Model file for the job. Use its own axes, mm. Face numbers are marked on the shaded views. A direction names the side the tool comes from. Coordinates: 2 decimals unless noted, no trailing zeros. Answer as a JSON object with one key per item and string values. Group by question number.
from build123d import *

# Parameters (mm, degrees)
F0_R     = 11
F1_DEPTH = 7
F2_R     = 3.4999


# Not quite as in the source:
# - a fillet or chamfer is up to 0.001 mm smaller than in the source, because OpenCascade refuses the exact size


with BuildPart() as f1:
    # F0 (on Front) → F1 (new body)
    with BuildSketch(Plane.XZ):
        with BuildLine():
            add(Edge.make_bspline(
                [(0, 31.75), (-29.1176115239, 31.75), (-14.558805762, -15.875), (0, -63.5), (14.558805762, -15.875), (29.1176115239, 31.75), (0, 31.75)],
                knots=[0, 0, 0, 2.0943951024, 2.0943951024, 4.1887902048, 4.1887902048, 6.2831853072, 6.2831853072, 6.2831853072], degree=2, weights=[1, 0.5, 1, 0.5, 1, 0.5, 1]))
        make_face()
        Polygon((2.9989406364, -15.1111775695), (6.0104428668, -20.3127475603), (3.0115022304, -25.5215699908), (-2.9989406364, -25.5288224305), (-6.0104428668, -20.3272524397), (-3.0115022304, -15.1184300092), align=None, mode=Mode.SUBTRACT)
        Circle(F0_R, mode=Mode.SUBTRACT)
        Polygon((2.9955036613, 25.5227137441), (6.0034341016, 20.3271746042), (3.0079304403, 15.1244608602), (-2.9955036613, 15.1172862559), (-6.0034341016, 20.3128253958), (-3.0079304403, 25.5155391398), align=None, mode=Mode.SUBTRACT)
    extrude(amount=F1_DEPTH)

    # F2 (radius 3.5 in the source; OpenCascade refuses exactly that, so slightly less here)
    f2_edges = [f1.edges().sort_by_distance(p)[0] for p in [
        (-2e-06, -7, -31.75),
        (-2e-06, 0, -31.75),
    ]]
    fillet(f2_edges, radius=F2_R)


solid = f1.part
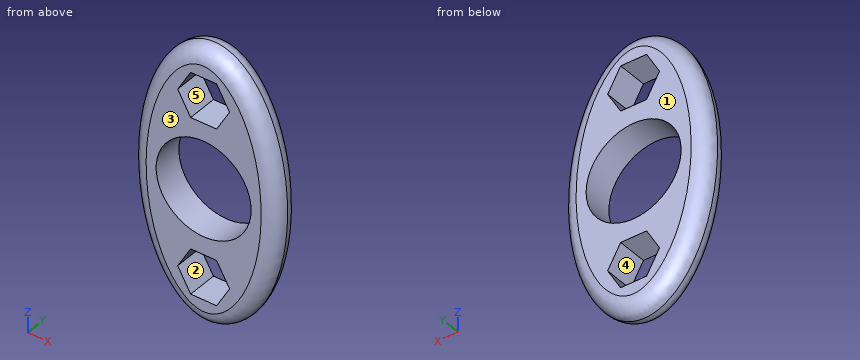
(1) Pin check, flat tip, straight feed: pin 1 (3 mm diameter, centred on x = -11, y = -6, fed in from +Z). Stop position of the tip, or through.
(2) Cut at A-A on y = -5.5. Give the number of separate pieces and of enclosed holes in the cut face, plus the area to 3 significant figures.
(3) Pull direction Z, two halves, no side cores. Call the marked faces 3, 4 and 5: released by +Z, released by -Z, zero draft, split by the parting line, or undercut.
(4) Wall check: probe 1 along Z at (x, y) = (0, -3.5); probe 2 along Z at (x, y) = (1.5, -5.5); probe 3 along Z at (x, y) = (-9, -3.5). Give the ranges that are in metal, low to high.
(5) 3-axis set-ups, long thin cutter, end or side, ignore diameter. For the marked faces 1 and 2: which of +Z, -Z, +X, -X, +Y, -Y reach the whole face in a straight line?
Results found:
{
 "1": {"pin 1": "stops at z = 25.14"},
 "2": {"separate pieces": "1", "enclosed holes": "3", "area": "1,010 mm²"},
 "3": {"face 3": "zero draft", "face 4": "undercut", "face 5": "undercut"},
 "4": {"probe 1": "z = -31.75 to -25.53, -15.11 to -11, 11 to 15.12, 25.52 to 31.75", "probe 2": "z = -30.99 to -25.52, -15.11 to -10.9, 10.9 to 15.12, 25.52 to 30.99", "probe 3": "z = -26.82 to -6.32, 6.32 to 26.82"},
 "5": {"face 1": "+Z, -Z, +X, -X, +Y", "face 2": "+Y, -Y"}
}
